For this review, take the finished solid that the model builds, in its own axes (mm). A direction names the side the tool comes from. Give positions to 0.01 mm unless a question says otherwise; leave off trailing zeros. Write each loop counter-clockwise with the first axis right and the second up, starting at its lowest first coordinate (ties: lowest second). Pieces come first, ordered by that corner, then holes.
1) We need section C-C on y = -1.25. Give the boundary of the cut face in (x, z).
2) We need section B-B on z = 12.75. Give the boundary of the cut face in (x, y), and give its area (3 significant figures).
3) Wall thickness on line 1 along Z through (x, y) = (-0.5, -1.5); line 2 along Y through (x, z) = (-1.75, 5); line 3 along Y through (x, z) = (2, 8.75): over which ranges is each line inside the solid? List them lowest first.
4) We need section A-A on x = 0. Give the boundary of the cut face in (y, z).
5) Machinability: for faces 1 (the face through (0.68, -3.22, 4.93)), 2 (the face through (0.63, -0.49, 15.42)), which of the approach directions +Z, -Z, +X, -X, +Y, -Y give a long, thin tool a straight path to every point of the face, cutting with its end or side? Answer none if there is none.
6) We need section D-D on z = 1.5. Give the boundary of the cut face in (x, y).
Autodesk Fusion 360 part; units mm, degrees
sketch "Sketch1" plane through (0, 0, 0) normal (0, 0, 1) x (1, 0, 0)
  line L0 (2.5647, -2.804) -> (3.7107, 0.819)
  line L1 (3.7107, 0.819) -> (1.146, 3.6231)
  line L2 (1.146, 3.6231) -> (-2.5647, 2.804)
  line L3 (-2.5647, 2.804) -> (-3.7107, -0.819)
  line L4 (-3.7107, -0.819) -> (-1.146, -3.6231)
  line L5 (-1.146, -3.6231) -> (2.5647, -2.804)
  dimension "d1" = 3.8
extrude "Extrude1" add sketch "Sketch1" along normal blind 10
sketch "Sketch2" plane through (0, 0, 10) normal (0, 0, 1) x (-1, 0, 0)
  line L0 (1.146, 3.6231) -> (-2.5647, 2.804)
  line L1 (-2.5647, 2.804) -> (-3.7107, -0.819)
  line L2 (-3.7107, -0.819) -> (-1.146, -3.6231)
  line L3 (-1.146, -3.6231) -> (2.5647, -2.804)
  line L4 (2.5647, -2.804) -> (3.7107, 0.819)
  line L5 (3.7107, 0.819) -> (1.146, 3.6231)
  circle A0 centre (0, 0) radius 0.8
  dimension "d6" = 1.6
extrude "Extrude2" add sketch "Sketch2" along normal blind 11 contours A0
equation "d1 = polygon_side"
equation "d2 = polygon_height"
equation "polygon_side = 3.8 mm"
equation "polygon_height = 10 mm"
equation "d6 = cylinder_radius * 2"
equation "cylinder_radius = 0.8 mm"
equation "cylinder_height = 11 mm"
equation "d9 = cylinder_height"
Results list:
1. outline: (-3.32, 0) - (3.06, 0) - (3.06, 10) - (-3.32, 10) - close
2. outline: circle Ø1.6 at (0, 0)
2. area: 2.01 mm2
3. line 1: z = 0 to 10
3. line 2: y = -2.96 to 2.98
3. line 3: y = -2.93 to 2.69
4. outline: (-3.37, 0) - (3.37, 0) - (3.37, 10) - (0.8, 10) - (0.8, 21) - (-0.8, 21) - (-0.8, 10) - (-3.37, 10) - close
5. face 1: +Z, -Z, +X, -Y
5. face 2: +Z
6. outline: (-3.71, -0.82) - (-1.15, -3.62) - (2.56, -2.8) - (3.71, 0.82) - (1.15, 3.62) - (-2.56, 2.8) - close
